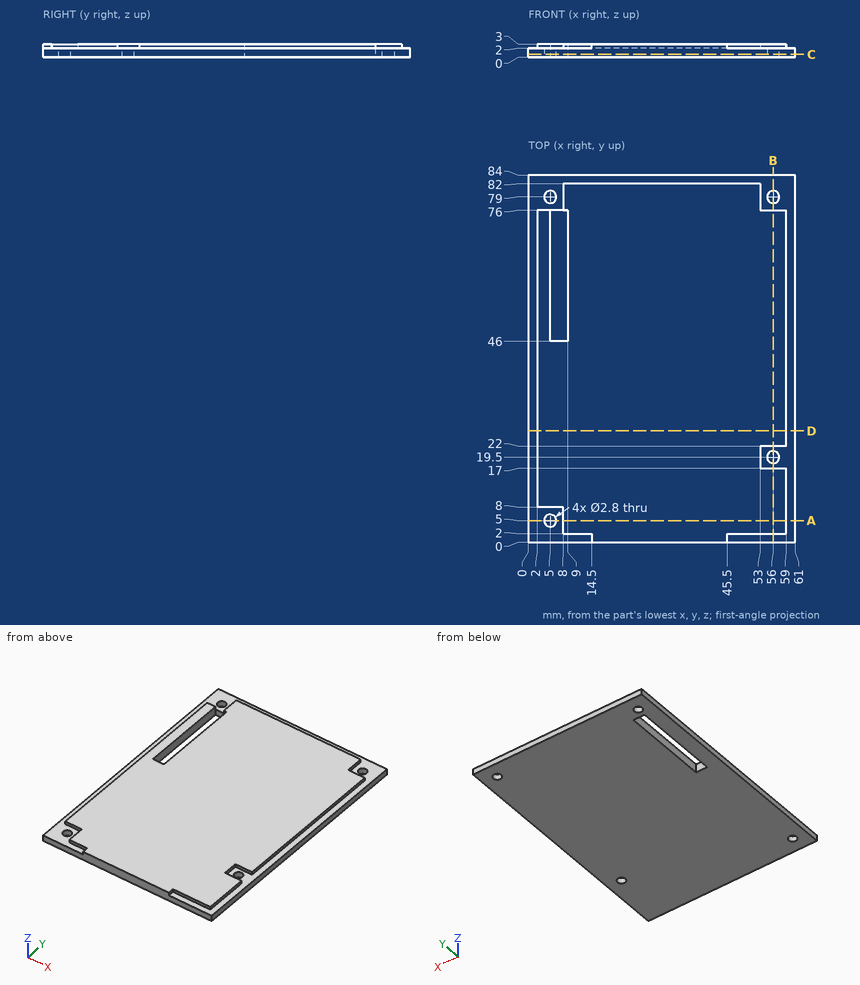
Here's the drawing with two shaded views (mm, measured from the low corner). I have some questions. Give positions to 0.01 mm unless a question says otherwise; leave off trailing zeros. Write each loop counter-clockwise with the first axis right and the second up, starting at its lowest first coordinate (ties: lowest second). Pieces come first, ordered by that corner, then holes. Notation, with made-up numbers: (8, -1) - (39, -1) arc R13 ccw to (39, 18) - close; hole circle Ø7 at (47, -18.5). An arc over 180 degrees is marked (long way). Write item = value, one per line. Start each with the question number.
1. Imagine slicing it at D-D (y = 25.5). Please give me the cut outline in (x, z).
2. Imagine slicing it at B-B (x = 56). Please give me the cut outline in (y, z), and give its area (3 significant figures).
3. For pin 1 (0.5 mm diameter, centred on x = 55.5, z = 2.5, fed in from +Y); pin 2 (0.5 mm diameter, centred on x = 55.5, z = 2.5, fed in from -Y); pin 3 (3.5 mm diameter, centred on x = 56, y = 19.5, fed in from +Z); pin 4 (1.1 mm diameter, centred on x = 55.5, z = 2.5, fed in from +Y), each with a flat end and sliding along its axis, tell me the tip position at first contact or that it passes through.
4. Imagine slicing it at C-C (z = 0.65). Please give me the cut outline in (x, y).
5. Please list where these lines run through material, in increasing order: line 1 (X direction, y = 79, z = 1.5); line 2 (Y direction, x = 56, z = 0.9); line 3 (X direction, y = 19.5, z = 1.3).
6. Imagine slicing it at A-A (y = 5). Please give me the cut outline in (x, z).
Worked answers:
q1.outline = (0, 0) - (61, 0) - (61, 2) - (59, 2) - (59, 3) - (2, 3) - (2, 2) - (0, 2) - close
q2.outline = (0, 0) - (18.1, 0) - (18.1, 2) - (17, 2) - (17, 3) - (2, 3) - (2, 2) - (0, 2) - close; (20.9, 0) - (77.6, 0) - (77.6, 2) - (76, 2) - (76, 3) - (22, 3) - (22, 2) - (20.9, 2) - close; (80.4, 0) - (84, 0) - (84, 2) - (80.4, 2) - close
q2.area = 226 mm2
q3.pin_1 = 76
q3.pin_2 = 2
q3.pin_3 = 2
q3.pin_4 = 84
q4.outline = (0, 0) - (61, 0) - (61, 84) - (0, 84) - close; hole circle Ø2.8 at (5, 5); hole circle Ø2.8 at (5, 79); hole (5, 46) - (9, 46) - (9, 76) - (5, 76) - close; hole circle Ø2.8 at (56, 19.5); hole circle Ø2.8 at (56, 79)
q5.line_1 = 0 to 3.6, 6.4 to 54.6, 57.4 to 61
q5.line_2 = 0 to 18.1, 20.9 to 77.6, 80.4 to 84
q5.line_3 = 0 to 54.6, 57.4 to 61
q6.outline = (0, 0) - (3.6, 0) - (3.6, 2) - (0, 2) - close; (6.4, 0) - (61, 0) - (61, 2) - (59, 2) - (59, 3) - (8, 3) - (8, 2) - (6.4, 2) - close
